Input: part model. Units: mm. Frame: model coordinates. Face numbers are marked on the shaded views. Round coordinates to 2 decimals unless told otherwise and drop trailing zeros. Use one line per item in the form item = value.
```python
from build123d import *

# Parameters (mm, degrees)
SKETCH1_R           = 31.75
BOSS_EXTRUDE1_DEPTH = 152.4
DRAFT1_ANGLE        = 4
SKETCH3_R           = 29.21
CUT_EXTRUDE1_DEPTH  = 3.175
SHELL2_T            = -2.54
SKETCH4_R           = 1.905


with BuildPart() as part:
    # Sketch1 → Boss-Extrude1 (new body)
    with BuildSketch(Plane(origin=(0, 0, 0), x_dir=(0, 0, -1), z_dir=(1, 0, 0))):
        with Locations(Location((0, 0, 0), (0, 0, 180))):
            Circle(SKETCH1_R)
    extrude(amount=BOSS_EXTRUDE1_DEPTH)

    # Draft1
    draft1_faces = [part.faces().sort_by_distance(p)[0] for p in [
        (76.2, 0, -31.75),
    ]]
    draft(draft1_faces, Plane(origin=(0, 0, 0), x_dir=(0, 0, -1), z_dir=(-1, 0, 0)), DRAFT1_ANGLE)

    # Sketch3 → Cut-Extrude1 (cut)
    with BuildSketch(Plane.ZY):
        Circle(SKETCH3_R)
    extrude(amount=-CUT_EXTRUDE1_DEPTH, mode=Mode.SUBTRACT)

    # Shell2
    shell2_openings = [part.faces().sort_by_distance(p)[0] for p in [
        (152.4, 0, 0),
    ]]
    offset(amount=SHELL2_T, openings=shell2_openings, kind=Kind.INTERSECTION)

    # Sketch4 → Revolve1 (revolve)
    with BuildSketch(Plane(origin=(0, 0, 0), x_dir=(1, 0, 0), z_dir=(0, 1, 0))):
        with Locations((152.4, 40.85216375)):
            Circle(SKETCH4_R)
    revolve(axis=Axis((152.4, 0, 0), (-1, 0, 0)))

    # Loft1: read off the stored shape, not the designer's step
    # Loft1: loft between two sections, ruled curve by curve
    loft1_from = [
        Edge.make_bspline([(5.715, 9.130270928, 28.160276626), (5.715, -47.190282323, 46.420818482), (5.715, -65.45082418, -9.89973477), (5.715, -9.130270928, -28.160276626), (5.715, 47.190282323, -46.420818482), (5.715, 65.45082418, 9.89973477), (5.715, 9.130270928, 28.160276626)], [0, 0, 0, 0, 0.5, 0.5, 0.5, 1, 1, 1, 1], 3, [1, 0.333333333, 0.333333333, 1, 0.333333333, 0.333333333, 1]),
    ]
    loft1_to = [
        Edge.make_bspline([(126.365, -16.699930799, 33.553520927), (126.365, -83.806972652, 0.153659328), (126.365, -50.407111054, -66.953382525), (126.365, 16.699930799, -33.553520927), (126.365, 83.806972652, -0.153659328), (126.365, 50.407111054, 66.953382525), (126.365, -16.699930799, 33.553520927)], [0, 0, 0, 0, 0.5, 0.5, 0.5, 1, 1, 1, 1], 3, [1, 0.333333333, 0.333333333, 1, 0.333333333, 0.333333333, 1]),
    ]
    loft1 = Solid(Shell([*[Face.make_surface_from_curves(loft1_from[k], loft1_to[k]) for k in range(1)], Face(Wire(loft1_from)), Face(Wire(loft1_to))]))
    add(loft1)


solid = part.part
```
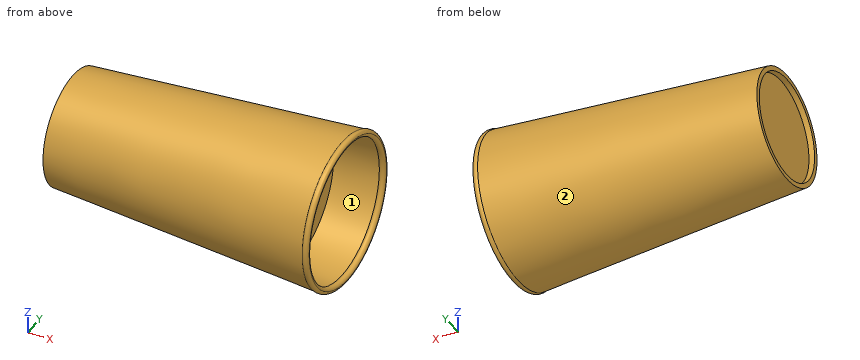
(1) First-contact query: pin 1 Ø12 at (x, y) = (127, -22.5) entering from +Z; pin 2 Ø1 at (x, y) = (87.5, -20.5) entering from +Z; pin 3 Ø22.5 at (y, z) = (1, -17.5) entering from +X (3 decimals). Flat tips, straight axial feed; report the tip coordinate or a pass-through.
Derived:
pin_1 = 37.17
pin_2 = 32.16
pin_3 = 126.365
(2) Cut plane A-A on x = 50.5. Count the separate pieces of the cut face and the enclosed holes in it, then the cut area to 3 significant figures.
Derived:
separate_pieces = 2
enclosed_holes = 1
area = 3,400 mm^2
(3) Material intervals for L1, parallel to Z at x = 59.5, y = -28; L2, parallel to Z at x = 71, y = -28; L3, parallel to Y at x = 84.5, z = 11.5, sorted ascending.
Derived:
L1 = -22.48 to -18.14, -12.49 to 12.49, 18.14 to 22.48
L2 = -23.75 to -19.58, -14.33 to 14.33, 19.58 to 23.75
L3 = -35.86 to -33.18, -30.52 to 30.52, 33.18 to 35.86
(4) Draft query along X for the marked faces 1 and 2. Return one class per face: released by +X, released by -X, zero draft, split by the parting line, or undercut.
Derived:
face_1 = undercut
face_2 = released by -X
